from build123d import *

# Parameters (mm, degrees)
F0_W      = 25.4
F0_H      = 50.8
F3_DEPTH  = 50.8
F1_W      = 25.4
F1_H      = 25.4
F4_DEPTH  = 50.8
F2_W      = 76.2
F2_H      = 25.4
F5_DEPTH  = 25.4
F5_FACE_W = 76.2
F5_FACE_H = 25.4
F6_DEPTH  = 25.4
F7_W      = 50.8
F7_H      = 25.4
F8_DEPTH  = 25.4


with BuildPart() as f3:
    # F0 (on Top) → F3 (new body)
    with BuildSketch(Plane.XY):
        with Locations((-12.7, -25.4)):
            Rectangle(F0_W, F0_H)
    extrude(amount=F3_DEPTH)

    # F1 (on Top) → F4 (join)
    with BuildSketch(Plane.XY):
        with Locations((-12.7, 12.7)):
            Rectangle(F1_W, F1_H)
    extrude(amount=F4_DEPTH)

    # F2 (on Top) → F5 (join)
    with BuildSketch(Plane.XY):
        with Locations((38.1, 12.7)):
            Rectangle(F2_W, F2_H)
    extrude(amount=F5_DEPTH)

    # F5_face (on face) → F6 (join)
    with BuildSketch(Plane(origin=(38.1, 12.7, 25.4), x_dir=(1, 0, 0), z_dir=(0, 0, 1))):
        Rectangle(F5_FACE_W, F5_FACE_H)
    extrude(amount=F6_DEPTH)

    # F7 (on Top) → F8 (join)
    with BuildSketch(Plane.XY):
        with Locations((101.3518, 12.7)):
            Rectangle(F7_W, F7_H)
    extrude(amount=F8_DEPTH)


solid = f3.part
Work out the finished part from the listing and answer in its coordinate system (mm). A direction names the side the tool comes from. Give positions to 0.01 mm unless a question says otherwise; leave off trailing zeros. Order: outer loops, then holes, each group sorted by start corner. A loop starts at its lowest first (then second) coordinate and runs counter-clockwise, first axis right, second up. Notation, with made-up numbers: (9, -30.75) -> (67, -30.75) arc R22 cw to (67, -24.75) -> close; hole circle Ø1 at (2.5, 69.5). An arc over 180 degrees is marked (long way). One line per item, written item: value.
Item 1: Find section A-A, the plane z = 17.5. Give the vertices of the cut face in (x, y), plus the area to 3 significant figures.
Answer sheet:
outline: (-25.4, -50.8) -> (0, -50.8) -> (0, 0) -> (126.75, 0) -> (126.75, 25.4) -> (-25.4, 25.4) -> close
area: 5,150 mm²
Item 2: Find section B-B, the plane y = 17.5. Give the vertices of the cut face in (x, z), plus the area to 3 significant figures.
Answer sheet:
outline: (-25.4, 0) -> (126.75, 0) -> (126.75, 25.4) -> (76.2, 25.4) -> (76.2, 50.8) -> (-25.4, 50.8) -> close
area: 6,450 mm²
Item 3: Flat-ended cylindrical pins translate along their axes: P1, Ø1.5, axis at y = -36, z = 13.5, coming from the +X side; P2, Ø20.5, axis at y = 13.5, z = 34.5, coming from the +X side; P3, Ø7.5, axis at x = 98, y = 19, coming from the +Z side; P4, Ø6, axis at x = 44.5, y = -5, coming from the +Z side. Find the tip coordinate at first contact, or state that the pin passes through.
Answer sheet:
P1: x = 0
P2: x = 126.75
P3: z = 25.4
P4: through
Item 4: Straight lines are drawn through the part: probe 1 along Y at (x, z) = (62, 5.5); probe 2 along X at (y, z) = (-32.5, 4.5). For each, find the intervals that lie inside material, in ascending order.
Answer sheet:
probe 1: 0 to 25.4
probe 2: -25.4 to 0
Item 5: Find section D-D, the plane y = -17.5. Give the vertices of the cut face in (x, z), plus the area to 3 significant figures.
Answer sheet:
outline: (-25.4, 0) -> (0, 0) -> (0, 50.8) -> (-25.4, 50.8) -> close
area: 1,290 mm²
Item 6: Find section C-C, the plane x = 14. Give the vertices of the cut face in (y, z), plus the area to 3 significant figures.
Answer sheet:
outline: (0, 0) -> (25.4, 0) -> (25.4, 50.8) -> (0, 50.8) -> close
area: 1,290 mm²
Item 7: A tool of negligible diameter and unlimited length cuts with its end or side. For faces 1 (the flat face through (48, 0, 19)), 2 (the flat face through (76.2, 13, 38)), 3 (the flat face through (-25.4, -13, 25)), from which of +Z, -Z, +X, -X, +Y, -Y can it reach the whole face along a straight path? Write none if from no direction.
Answer sheet:
face 1: +Z, -Z, +X, -Y
face 2: +Z, +X, +Y, -Y
face 3: +Z, -Z, -X, +Y, -Y
